Input: part model. Units: mm. Frame: model coordinates. Face numbers are marked on the shaded views. A direction names the side the tool comes from. Give positions to 0.01 mm unless a question says otherwise; leave off trailing zeros. Loops run counter-clockwise (first coordinate to the right, second up) from the corner with the lowest first, then second, coordinate; pieces in that order, holes last. Notation, with made-up numbers: M 31,25 L 36,25 A28 ccw 36,43 Z; hole C 4,-22.75 d9. An arc over 180 degrees is marked long. One line per item, written item: value. Start each with the question number.
(1) Section C-C on z = 126. Output: boundary loops of the cut face in (x, y), plus the area to 3 significant figures.
(2) Ray query, line 1 along Y through (x, z) = (0, 3.75); line 2 along Z through (x, y) = (19, -2); line 3 along X through (y, z) = (18, 0.5). Return the intervals inside material, ascending. Write a range as from..to.
(3) Access query for the marked faces 1, 2 and 3. Directions: +Z, -Z, +X, -X, +Y, -Y. A direction counts if a zero-diameter tool reaches every point of the face in a straight line with its end or side. Return the directions, or none.
(4) Pin query (flat end, axial travel): P1, Ø1, axis at x = 6.5, y = 1, coming from the +Z side; P2, Ø4, axis at x = -29, y = -38.5, coming from the +Z side; P3, Ø6, axis at x = -6, z = 139.5, coming from the -Y side. Return the tip coordinate at first contact, or that it passes through.
(5) Section A-A on y = 0. Output: boundary loops of the cut face in (x, z).
(6) Section B-B on x = 24.5. Output: boundary loops of the cut face in (y, z), plus the area to 3 significant figures.
(7) Section D-D on y = -28. Output: boundary loops of the cut face in (x, z), plus the area to 3 significant figures.
```python
from build123d import *

# Parameters (mm, degrees)
SKETCH1_R           = 50.8
BOSS_EXTRUDE1_DEPTH = 250
SKETCH2_R           = 47.5
CUT_EXTRUDE1_DEPTH  = 5
CUT_EXTRUDE2_START  = -5
SKETCH3_R           = 47.5
CUT_EXTRUDE2_DEPTH  = 5
SKETCH4_R           = 8
BOSS_EXTRUDE2_DEPTH = 15
BOSS_EXTRUDE3_START = 15
SKETCH5_R           = 8
BOSS_EXTRUDE3_DEPTH = 15
SKETCH7_R           = 6
BOSS_EXTRUDE4_DEPTH = 10
BOSS_EXTRUDE5_START = 10
SKETCH8_R           = 6
BOSS_EXTRUDE5_DEPTH = 10


with BuildPart() as part:
    # Sketch1 → Boss-Extrude1 (new body)
    with BuildSketch(Plane.XY):
        Circle(SKETCH1_R)
    extrude(amount=BOSS_EXTRUDE1_DEPTH)

    # Sketch2 → Cut-Extrude1 (cut)
    with BuildSketch(Plane.XY.offset(250)):
        Circle(SKETCH2_R)
    extrude(amount=-CUT_EXTRUDE1_DEPTH, mode=Mode.SUBTRACT)

    # Sketch3 → Cut-Extrude2 (cut)
    with BuildSketch(Plane(origin=(0, 0, 0), x_dir=(-1, 0, 0), z_dir=(0, 0, -1)).offset(CUT_EXTRUDE2_START)):
        with Locations(Location((0, 0, 0), (0, 0, 180))):
            Circle(SKETCH3_R)
    extrude(amount=CUT_EXTRUDE2_DEPTH, mode=Mode.SUBTRACT)

    # Sketch4 → Boss-Extrude2 (add)
    with BuildSketch(Plane(origin=(0, 0, 5), x_dir=(-1, 0, 0), z_dir=(0, 0, -1))):
        Circle(SKETCH4_R)
    extrude(amount=BOSS_EXTRUDE2_DEPTH)

    # Sketch5 → Boss-Extrude3 (add)
    with BuildSketch(Plane.XY.offset(245).offset(BOSS_EXTRUDE3_START)):
        with Locations(Location((0, 0, 0), (0, 0, 180))):
            Circle(SKETCH5_R)
    extrude(amount=-BOSS_EXTRUDE3_DEPTH)

    # Sketch7 → Boss-Extrude4 (add)
    with BuildSketch(Plane(origin=(0, 0, -10), x_dir=(-1, 0, 0), z_dir=(0, 0, -1))):
        Circle(SKETCH7_R)
    extrude(amount=BOSS_EXTRUDE4_DEPTH)

    # Sketch8 → Boss-Extrude5 (add)
    with BuildSketch(Plane.XY.offset(260).offset(BOSS_EXTRUDE5_START)):
        with Locations(Location((0, 0, 0), (0, 0, 180))):
            Circle(SKETCH8_R)
    extrude(amount=-BOSS_EXTRUDE5_DEPTH)


solid = part.part
```
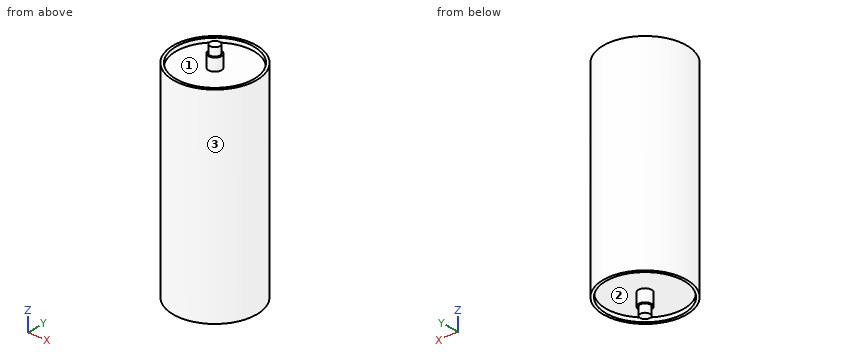
Output values:
1. outline: C 0,0 d101.6
1. area: 8,110 mm²
2. line 1: y = -50.8..-47.5, -8..8, 47.5..50.8
2. line 2: z = 5..245
2. line 3: x = -47.5..-43.96, 43.96..47.5
3. face 1: +Z
3. face 2: -Z
3. face 3: +Z, -Z
4. P1: stops at z = 260
4. P2: stops at z = 250
4. P3: stops at y = -50.71
5. outline: M -50.8,0 L -47.5,0 L -47.5,5 L -8,5 L -8,-10 L -6,-10 L -6,-20 L 6,-20 L 6,-10 L 8,-10 L 8,5 L 47.5,5 L 47.5,0 L 50.8,0 L 50.8,250 L 47.5,250 L 47.5,245 L 8,245 L 8,260 L 6,260 L 6,270 L -6,270 L -6,260 L -8,260 L -8,245 L -47.5,245 L -47.5,250 L -50.8,250 Z
6. outline: M -44.5,0 L -40.69,0 L -40.69,5 L 40.69,5 L 40.69,0 L 44.5,0 L 44.5,250 L 40.69,250 L 40.69,245 L -40.69,245 L -40.69,250 L -44.5,250 Z
6. area: 21,400 mm²
7. outline: M -42.39,0 L -38.37,0 L -38.37,5 L 38.37,5 L 38.37,0 L 42.39,0 L 42.39,250 L 38.37,250 L 38.37,245 L -38.37,245 L -38.37,250 L -42.39,250 Z
7. area: 20,400 mm²
